Read the model definition and answer for the solid it produces. Units are mm, in the model's axes. Face numbers are marked on the shaded views. Round coordinates to 2 decimals unless told otherwise and drop trailing zeros. Use CSV: the item, a comma, the result in double quotes. Start each with the question number.
1. Determine the mould class of the marked faces 1 and 2 for opening direction Z: +Z half, -Z half, draft (parallel to the pull), parting line (faces both ways), or undercut.
2. Given pin 1 Ø6 at (x, y) = (24.5, -101.5) entering from -Z; pin 2 Ø4 at (x, z) = (-20, 5) entering from +Y; pin 3 Ø3 at (x, z) = (20, 5) entering from +Y, each flat-ended and moving along its own axis, determine where each tip first touches the part or whether it passes through.
3. Consider line 1 along X through (y, z) = (-136.25, 5); line 2 along Z through (x, y) = (-20, 136.25); line 3 along Y through (x, z) = (19, 4.75). Determine where each line is inside the solid, lowest interval first.
from build123d import *

# Parameters (mm, degrees)
F0_W     = 65
F0_H     = 280
F1_DEPTH = 10
F4_D     = 5
F4_DEPTH = 12
F4_TIP   = 1.5021515476
F7_D     = 5
F7_DEPTH = 12
F7_TIP   = 1.5021515476


with BuildPart() as f1:
    # F0 (on Top) → F1 (new body)
    with BuildSketch(Plane.XY):
        Rectangle(F0_W, F0_H)
    extrude(amount=F1_DEPTH)

    # F4
    with Locations(Plane.XZ.offset(140)):
        with Locations((-22, 5), (20, 5)):
            Hole(F4_D / 2, depth=F4_DEPTH)
            with Locations((0, 0, -(F4_DEPTH + F4_TIP / 2))):  # 118° drill point
                Cone(0, F4_D / 2, F4_TIP, mode=Mode.SUBTRACT)

    # F7
    with Locations(Plane(origin=(0, 140, 0), x_dir=(1, 0, 0), z_dir=(0, 1, 0))):
        with Locations((-20, -5), (20, -5)):
            Hole(F7_D / 2, depth=F7_DEPTH)
            with Locations((0, 0, -(F7_DEPTH + F7_TIP / 2))):  # 118° drill point
                Cone(0, F7_D / 2, F7_TIP, mode=Mode.SUBTRACT)


solid = f1.part
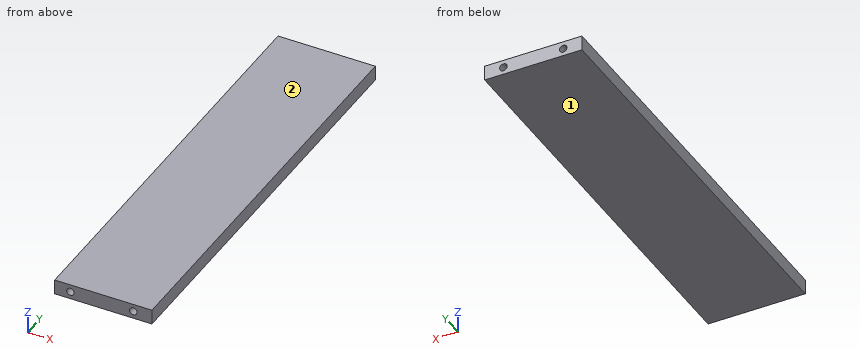
Filled sheet:
1,face 1,"-Z half"
1,face 2,"+Z half"
2,pin 1,"stops at z = 0"
2,pin 2,"stops at y = 127.7"
2,pin 3,"stops at y = 127.4"
3,line 1,"x = -32.5 to -24.5, -19.5 to 17.5, 22.5 to 32.5"
3,line 2,"z = 0 to 2.5, 7.5 to 10"
3,line 3,"y = -127.12 to 127.12"
